from build123d import *

# Parameters (mm, degrees)
SKETCH_1_W                = 56.3
SKETCH_1_H                = 39
SKETCH_1_R                = 1
EXTRUDE_1_DEPTH           = 1.5
SKETCH_2_W                = 46.047970844
SKETCH_2_H                = 34
EXTRUDE_2_DEPTH           = 2.25
SKETCH_3_W                = 35.04
SKETCH_3_H                = 28.03
CUT_EXTRUDE_1_DEPTH       = 0.1
SKETCH_5_R                = 1
EXTRUDE_4_DEPTH           = 2
EXTRUDE_4_DRAFT           = 15
EXTRUDE_4_PROFILE_2_DEPTH = 2
EXTRUDE_4_PROFILE_2_DRAFT = 15
EXTRUDE_4_PROFILE_3_DEPTH = 2
EXTRUDE_4_PROFILE_3_DRAFT = 15
EXTRUDE_4_PROFILE_4_DEPTH = 2
EXTRUDE_4_PROFILE_4_DRAFT = 15
EXTRUDE_4_PROFILE_5_DEPTH = 2
EXTRUDE_4_PROFILE_5_DRAFT = 15
EXTRUDE_4_PROFILE_6_DEPTH = 2
EXTRUDE_4_PROFILE_6_DRAFT = 15
EXTRUDE_4_PROFILE_7_DEPTH = 2
EXTRUDE_4_PROFILE_7_DRAFT = 15
EXTRUDE_4_PROFILE_8_DEPTH = 2
EXTRUDE_4_PROFILE_8_DRAFT = 15


with BuildPart() as part:
    # Эскиз1 → Бобышка-Вытянуть1 (new body)
    with BuildSketch(Plane(origin=(0, 0, 0), x_dir=(1, 0, 0), z_dir=(0, 1, 0))):
        with Locations((-2.63, -1.52)):
            Rectangle(SKETCH_1_W, SKETCH_1_H)
        with Locations(Location((-28.48, 15.68, 0), (0, 0, 270))):
            Circle(SKETCH_1_R, mode=Mode.SUBTRACT)
        with Locations(Location((23.22, 15.68, 0), (0, 0, 270))):
            Circle(SKETCH_1_R, mode=Mode.SUBTRACT)
        with Locations(Location((-28.48, -18.72, 0), (0, 0, 270))):
            Circle(SKETCH_1_R, mode=Mode.SUBTRACT)
        with Locations(Location((23.22, -18.72, 0), (0, 0, 270))):
            Circle(SKETCH_1_R, mode=Mode.SUBTRACT)
    extrude(amount=EXTRUDE_1_DEPTH)

    # Эскиз2 → Бобышка-Вытянуть2 (add)
    with BuildSketch(Plane(origin=(0, 1.5, 0), x_dir=(1, 0, 0), z_dir=(0, 1, 0))):
        with Locations((-2.673985422, -1.52)):
            Rectangle(SKETCH_2_W, SKETCH_2_H)
    extrude(amount=EXTRUDE_2_DEPTH)

    # Эскиз3 → Вырез-Вытянуть1 (cut)
    with BuildSketch(Plane(origin=(0, 3.75, 0), x_dir=(1, 0, 0), z_dir=(0, 1, 0))):
        with Locations((0, -1.52)):
            Rectangle(SKETCH_3_W, SKETCH_3_H)
    extrude(amount=-CUT_EXTRUDE_1_DEPTH, mode=Mode.SUBTRACT)


with BuildPart() as extrude_4_tool:
    # Эскиз5 → Бобышка-Вытянуть4 (with draft: the straight prism first)
    with BuildSketch(Plane(origin=(0, 1.5, 0), x_dir=(1, 0, 0), z_dir=(0, 1, 0))):
        with Locations((22.99, 12.26)):
            Circle(SKETCH_5_R)
    extrude(amount=EXTRUDE_4_DEPTH)
    # Бобышка-Вытянуть4: the draft: its side faces are tilted about the plane it starts from
    extrude_4_sides = [extrude_4_tool.faces().sort_by_distance(p)[0] for p in [
        (21.99, 2.5, -12.26),
    ]]
    draft(extrude_4_sides, Plane(origin=(0, 1.5, 0), x_dir=(1, 0, 0), z_dir=(0, 1, 0)), EXTRUDE_4_DRAFT)


with BuildPart() as part_1:
    add(part.part)

    # Бобышка-Вытянуть4: add extrude_4_tool
    add(extrude_4_tool.part)


with BuildPart() as extrude_4_profile_2_tool:
    # Эскиз5 → Бобышка-Вытянуть4 profile 2 (with draft: the straight prism first)
    with BuildSketch(Plane(origin=(0, 1.5, 0), x_dir=(1, 0, 0), z_dir=(0, 1, 0))):
        with Locations((22.99, 9.72)):
            Circle(SKETCH_5_R)
    extrude(amount=EXTRUDE_4_PROFILE_2_DEPTH)
    # Бобышка-Вытянуть4 profile 2: the draft: its side faces are tilted about the plane it starts from
    extrude_4_profile_2_sides = [extrude_4_profile_2_tool.faces().sort_by_distance(p)[0] for p in [
        (21.99, 2.5, -9.72),
    ]]
    draft(extrude_4_profile_2_sides, Plane(origin=(0, 1.5, 0), x_dir=(1, 0, 0), z_dir=(0, 1, 0)), EXTRUDE_4_PROFILE_2_DRAFT)


with BuildPart() as part_2:
    add(part_1.part)

    # Бобышка-Вытянуть4 profile 2: add extrude_4_profile_2_tool
    add(extrude_4_profile_2_tool.part)


with BuildPart() as extrude_4_profile_3_tool:
    # Эскиз5 → Бобышка-Вытянуть4 profile 3 (with draft: the straight prism first)
    with BuildSketch(Plane(origin=(0, 1.5, 0), x_dir=(1, 0, 0), z_dir=(0, 1, 0))):
        with Locations((22.99, 7.18)):
            Circle(SKETCH_5_R)
    extrude(amount=EXTRUDE_4_PROFILE_3_DEPTH)
    # Бобышка-Вытянуть4 profile 3: the draft: its side faces are tilted about the plane it starts from
    extrude_4_profile_3_sides = [extrude_4_profile_3_tool.faces().sort_by_distance(p)[0] for p in [
        (21.99, 2.5, -7.18),
    ]]
    draft(extrude_4_profile_3_sides, Plane(origin=(0, 1.5, 0), x_dir=(1, 0, 0), z_dir=(0, 1, 0)), EXTRUDE_4_PROFILE_3_DRAFT)


with BuildPart() as part_3:
    add(part_2.part)

    # Бобышка-Вытянуть4 profile 3: add extrude_4_profile_3_tool
    add(extrude_4_profile_3_tool.part)


with BuildPart() as extrude_4_profile_4_tool:
    # Эскиз5 → Бобышка-Вытянуть4 profile 4 (with draft: the straight prism first)
    with BuildSketch(Plane(origin=(0, 1.5, 0), x_dir=(1, 0, 0), z_dir=(0, 1, 0))):
        with Locations((22.99, 4.64)):
            Circle(SKETCH_5_R)
    extrude(amount=EXTRUDE_4_PROFILE_4_DEPTH)
    # Бобышка-Вытянуть4 profile 4: the draft: its side faces are tilted about the plane it starts from
    extrude_4_profile_4_sides = [extrude_4_profile_4_tool.faces().sort_by_distance(p)[0] for p in [
        (21.99, 2.5, -4.64),
    ]]
    draft(extrude_4_profile_4_sides, Plane(origin=(0, 1.5, 0), x_dir=(1, 0, 0), z_dir=(0, 1, 0)), EXTRUDE_4_PROFILE_4_DRAFT)


with BuildPart() as part_4:
    add(part_3.part)

    # Бобышка-Вытянуть4 profile 4: add extrude_4_profile_4_tool
    add(extrude_4_profile_4_tool.part)


with BuildPart() as extrude_4_profile_5_tool:
    # Эскиз5 → Бобышка-Вытянуть4 profile 5 (with draft: the straight prism first)
    with BuildSketch(Plane(origin=(0, 1.5, 0), x_dir=(1, 0, 0), z_dir=(0, 1, 0))):
        with Locations((22.99, 2.1)):
            Circle(SKETCH_5_R)
    extrude(amount=EXTRUDE_4_PROFILE_5_DEPTH)
    # Бобышка-Вытянуть4 profile 5: the draft: its side faces are tilted about the plane it starts from
    extrude_4_profile_5_sides = [extrude_4_profile_5_tool.faces().sort_by_distance(p)[0] for p in [
        (21.99, 2.5, -2.1),
    ]]
    draft(extrude_4_profile_5_sides, Plane(origin=(0, 1.5, 0), x_dir=(1, 0, 0), z_dir=(0, 1, 0)), EXTRUDE_4_PROFILE_5_DRAFT)


with BuildPart() as part_5:
    add(part_4.part)

    # Бобышка-Вытянуть4 profile 5: add extrude_4_profile_5_tool
    add(extrude_4_profile_5_tool.part)


with BuildPart() as extrude_4_profile_6_tool:
    # Эскиз5 → Бобышка-Вытянуть4 profile 6 (with draft: the straight prism first)
    with BuildSketch(Plane(origin=(0, 1.5, 0), x_dir=(1, 0, 0), z_dir=(0, 1, 0))):
        with Locations((22.99, -0.44)):
            Circle(SKETCH_5_R)
    extrude(amount=EXTRUDE_4_PROFILE_6_DEPTH)
    # Бобышка-Вытянуть4 profile 6: the draft: its side faces are tilted about the plane it starts from
    extrude_4_profile_6_sides = [extrude_4_profile_6_tool.faces().sort_by_distance(p)[0] for p in [
        (21.99, 2.5, 0.44),
    ]]
    draft(extrude_4_profile_6_sides, Plane(origin=(0, 1.5, 0), x_dir=(1, 0, 0), z_dir=(0, 1, 0)), EXTRUDE_4_PROFILE_6_DRAFT)


with BuildPart() as part_6:
    add(part_5.part)

    # Бобышка-Вытянуть4 profile 6: add extrude_4_profile_6_tool
    add(extrude_4_profile_6_tool.part)


with BuildPart() as extrude_4_profile_7_tool:
    # Эскиз5 → Бобышка-Вытянуть4 profile 7 (with draft: the straight prism first)
    with BuildSketch(Plane(origin=(0, 1.5, 0), x_dir=(1, 0, 0), z_dir=(0, 1, 0))):
        with Locations((22.99, -2.98)):
            Circle(SKETCH_5_R)
    extrude(amount=EXTRUDE_4_PROFILE_7_DEPTH)
    # Бобышка-Вытянуть4 profile 7: the draft: its side faces are tilted about the plane it starts from
    extrude_4_profile_7_sides = [extrude_4_profile_7_tool.faces().sort_by_distance(p)[0] for p in [
        (21.99, 2.5, 2.98),
    ]]
    draft(extrude_4_profile_7_sides, Plane(origin=(0, 1.5, 0), x_dir=(1, 0, 0), z_dir=(0, 1, 0)), EXTRUDE_4_PROFILE_7_DRAFT)


with BuildPart() as part_7:
    add(part_6.part)

    # Бобышка-Вытянуть4 profile 7: add extrude_4_profile_7_tool
    add(extrude_4_profile_7_tool.part)


with BuildPart() as extrude_4_profile_8_tool:
    # Эскиз5 → Бобышка-Вытянуть4 profile 8 (with draft: the straight prism first)
    with BuildSketch(Plane(origin=(0, 1.5, 0), x_dir=(1, 0, 0), z_dir=(0, 1, 0))):
        with Locations((22.99, -5.52)):
            Circle(SKETCH_5_R)
    extrude(amount=EXTRUDE_4_PROFILE_8_DEPTH)
    # Бобышка-Вытянуть4 profile 8: the draft: its side faces are tilted about the plane it starts from
    extrude_4_profile_8_sides = [extrude_4_profile_8_tool.faces().sort_by_distance(p)[0] for p in [
        (21.99, 2.5, 5.52),
    ]]
    draft(extrude_4_profile_8_sides, Plane(origin=(0, 1.5, 0), x_dir=(1, 0, 0), z_dir=(0, 1, 0)), EXTRUDE_4_PROFILE_8_DRAFT)


with BuildPart() as part_8:
    add(part_7.part)

    # Бобышка-Вытянуть4 profile 8: add extrude_4_profile_8_tool
    add(extrude_4_profile_8_tool.part)


solid = part_8.part
Geometry check sheet. Reference: the model listing, model coordinates, mm. A direction names the side the tool comes from. Give positions to 0.01 mm unless a question says otherwise; leave off trailing zeros. Order: outer loops, then holes, each group sorted by start corner. A loop starts at its lowest first (then second) coordinate and runs counter-clockwise, first axis right, second up.
1) Cross-section at D-D (x = -23). Record the boundary of the cut face in (y, z).
Results are:
outline: (0, -17.98) - (1.5, -17.98) - (1.5, -15.48) - (3.75, -15.48) - (3.75, 18.52) - (1.5, 18.52) - (1.5, 21.02) - (0, 21.02) - close
2) Tool access check on faces 4 (the cylindrical face through (-28.44, 0.74, -16.68)), 5 (the flat face through (20.35, 3, 2)), 6 (the flat face through (-7, 1.5, -16)). Record the directions out of +Z, -Z, +X, -X, +Y, -Y that give a thin tool (end or side, any length) a straight path to the whole face; none if there is none.
Results are:
face 4: +Y, -Y
face 5: +Z, -Z, +Y
face 6: +Y
3) Draft check along Z on faces 1 (the flat face through (25.52, 1, 2)), 2 (the flat face through (-3, 1, 21.02)), 3 (the conical face through (23.615, 2.708, -9.461)). Enter one of: released by +Z, released by -Z, zero draft, split by the parting line, or undercut.
Results are:
face 1: zero draft
face 2: released by +Z
face 3: undercut
4) Cross-section at A-A (x = -12). Record the boundary of the cut face in (y, z) (3 decimals).
Results are:
outline: (0, -17.98) - (1.5, -17.98) - (1.5, -15.48) - (3.75, -15.48) - (3.75, -12.495) - (3.65, -12.495) - (3.65, 15.535) - (3.75, 15.535) - (3.75, 18.52) - (1.5, 18.52) - (1.5, 21.02) - (0, 21.02) - close
5) Gauge pin test, flat ends, axial feed: pin 1 (0.7 mm diameter, centred on x = -11, y = 2, fed in from -Z); pin 2 (0.7 mm diameter, centred on y = 2, z = -3, fed in from -X); pin 3 (0.7 mm diameter, centred on x = 23, z = -2.5, fed in from +Y). Record the tip position at first contact, or that the pin passes through.
Results are:
pin 1: stops at z = -15.48
pin 2: stops at x = -25.7
pin 3: stops at y = 3.5
6) Cross-section at C-C (y = 2.5). Give the number of separate pieces and of enclosed holes in the cut face, then the cut area to 3 significant figures.
Results are:
separate pieces: 9
enclosed holes: 0
area: 1,580 mm2
7) Material ranges on probe 1 along X at (y, z) = (0.45, 18.72); probe 2 along X at (y, z) = (0.25, -16); probe 3 along Y at (x, z) = (-13.5, -9.5), recorded low to high.
Results are:
probe 1: x = -30.78 to -29.48, -27.48 to 22.22, 24.22 to 25.52
probe 2: x = -30.78 to -29.43, -27.53 to 22.27, 24.17 to 25.52
probe 3: y = 0 to 3.65
8) Cross-section at B-B (z = -14). Record the boundary of the cut face in (x, y), then the cut area to 3 significant figures.
Results are:
outline: (-30.78, 0) - (25.52, 0) - (25.52, 1.5) - (20.35, 1.5) - (20.35, 3.75) - (-25.7, 3.75) - (-25.7, 1.5) - (-30.78, 1.5) - close
area: 188 mm2
